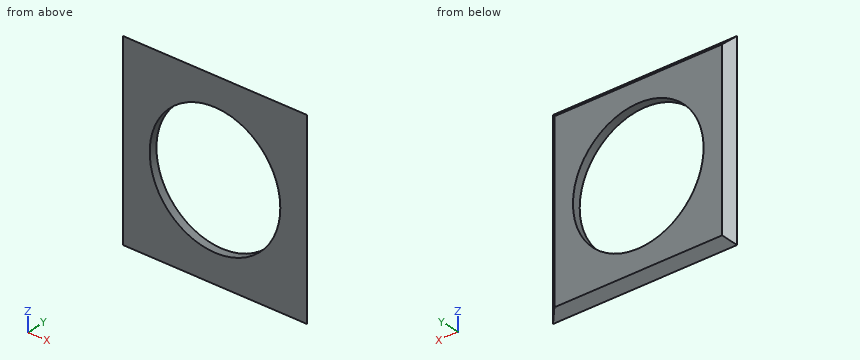
from build123d import *

# Parameters (mm, degrees)
F0_W     = 500
F0_H     = 510
F0_R     = 177.5
F1_DEPTH = 22
F2_SIZE  = 21.99999


# Not quite as in the source:
# - a fillet or chamfer is up to 0.001 mm smaller than in the source, because OpenCascade refuses the exact size


with BuildPart() as f1:
    # F0 (on Front) → F1 (new body)
    with BuildSketch(Plane.XZ):
        Rectangle(F0_W, F0_H)
        with BuildLine():
            Line((-161.5, 206.5), (161.5, 206.5))
            ThreePointArc((161.5, 206.5), (189.7842712475, 194.7842712475), (201.5, 166.5))
            Line((201.5, 166.5), (201.5, -166.5))
            ThreePointArc((201.5, -166.5), (189.7842712475, -194.7842712475), (161.5, -206.5))
            Line((161.5, -206.5), (-161.5, -206.5))
            ThreePointArc((-161.5, -206.5), (-189.7842712475, -194.7842712475), (-201.5, -166.5))
            Line((-201.5, -166.5), (-201.5, 166.5))
            ThreePointArc((-201.5, 166.5), (-189.7842712475, 194.7842712475), (-161.5, 206.5))
        make_face(mode=Mode.SUBTRACT)
        with BuildLine():
            ThreePointArc((201.5, 166.5), (189.7842712475, 194.7842712475), (161.5, 206.5))
            Line((161.5, 206.5), (-161.5, 206.5))
            ThreePointArc((-161.5, 206.5), (-189.7842712475, 194.7842712475), (-201.5, 166.5))
            Line((-201.5, 166.5), (-201.5, -166.5))
            ThreePointArc((-201.5, -166.5), (-189.7842712475, -194.7842712475), (-161.5, -206.5))
            Line((-161.5, -206.5), (161.5, -206.5))
            ThreePointArc((161.5, -206.5), (189.7842712475, -194.7842712475), (201.5, -166.5))
            Line((201.5, -166.5), (201.5, 166.5))
        make_face()
        Circle(F0_R, mode=Mode.SUBTRACT)
    extrude(amount=F1_DEPTH)

    # F2 (size 22 in the source; OpenCascade refuses exactly that, so slightly less here)
    f2_edges = [f1.edges().sort_by_distance(p)[0] for p in [
        (0, 0, 255),
        (250, 0, 0),
        (0, 0, -255),
        (-250, 0, 0),
    ]]
    chamfer(f2_edges, length=F2_SIZE)


solid = f1.part
Check sheet for the modelled part. Datum: model origin and axes. Units: mm. Give positions to 0.01 mm unless a question says otherwise; leave off trailing zeros. Write each loop counter-clockwise with the first axis right and the second up, starting at its lowest first coordinate (ties: lowest second). Pieces come first, ordered by that corner, then holes. Notation, with made-up numbers: (-34.75, 17.5) -> (18.25, 17.5) arc R31 ccw to (18.25, 42.5) -> close; hole circle Ø11 at (87, 51.25). An arc over 180 degrees is marked (long way). One line per item, written item: value. Start each with the question number.
Item 1: Gauge pin test, flat ends, axial feed: pin 1 (1 mm diameter, centred on y = -16.5, z = 121, fed in from -X); pin 2 (12 mm diameter, centred on y = -15, z = 119, fed in from -X); pin 3 (1 mm diameter, centred on x = 16, y = -18, fed in from +Z). Record the tip position at first contact, or that the pin passes through.
Item 2: Material ranges on probe 1 along Z at (x, y) = (116, -14.5); probe 2 along Z at (x, y) = (0, -10); probe 3 along X at (y, z) = (-13.5, -135.5), recorded low to high. Write a range as from..to.
Item 3: Section check C-C on y = -8.25. Record the cut outline in (x, z), then the cut area to 3 significant figures.
Results list:
1. pin 1: x = -245
1. pin 2: x = -249
1. pin 3: z = 251.5
2. probe 1: -247.5..-134.35, 134.35..247.5
2. probe 2: -243..-177.5, 177.5..243
2. probe 3: -241.5..-114.66, 114.66..241.5
3. outline: (-236.25, -241.25) -> (236.25, -241.25) -> (236.25, 241.25) -> (-236.25, 241.25) -> close; hole circle Ø355 at (0, 0)
3. area: 129,000 mm²
